```python
from build123d import *

# Parameters (mm, degrees)
SKETCH1_R                = 28.5
BOSS_EXTRUDE1_DEPTH      = 3
BOSS_EXTRUDE4_DEPTH      = 20
BOSS_EXTRUDE7_DEPTH      = 3
SKETCH7_R                = 27
SKETCH7_R_2              = 25
CUT_EXTRUDE1_DEPTH       = 3
CUT_EXTRUDE2_START       = -5
CUT_EXTRUDE2_DEPTH       = 5
CUT_EXTRUDE3_START       = -5
CUT_EXTRUDE3_DEPTH       = 5
BOSS_EXTRUDE8_DEPTH      = 2
BOSS_EXTRUDE8_DEPTH_BACK = 0.5
SKETCH10_R               = 26.875
CHAMFER1_SIZE            = 13.49895933
BOSS_EXTRUDE9_START      = 8
SKETCH11_R               = 26.875
SKETCH11_R_2             = 25.125
BOSS_EXTRUDE9_DEPTH      = 8
CUT_EXTRUDE4_START       = -2
CUT_EXTRUDE4_DEPTH       = 2
SKETCH12_R               = 5
BOSS_EXTRUDE10_DEPTH     = 6
CUT_EXTRUDE5_DEPTH       = 6


with BuildPart() as part:
    # Sketch1 → Boss-Extrude1 (new body)
    with BuildSketch(Plane(origin=(0, 0, 0), x_dir=(1, 0, 0), z_dir=(0, 1, 0))):
        with Locations(Location((0, 0, 0), (0, 0, 270))):
            Circle(SKETCH1_R)
    extrude(amount=BOSS_EXTRUDE1_DEPTH)

    # Sketch2 → Boss-Extrude4 (add)
    with BuildSketch(Plane(origin=(0, 3, 0), x_dir=(1, 0, 0), z_dir=(0, 1, 0))):
        with BuildLine():
            Line((-9, -20.223805295), (-9, -18.723805295))
            ThreePointArc((-9, -18.723805295), (-11.855740218, -15.445899804), (-13.568253388, -11.45))
            ThreePointArc((-13.568253388, -11.45), (-14, -8), (-13.568253388, -4.55))
            ThreePointArc((-13.568253388, -4.55), (0, 6), (13.568253388, -4.55))
            ThreePointArc((13.568253388, -4.55), (14, -8), (13.568253388, -11.45))
            ThreePointArc((13.568253388, -11.45), (11.855740218, -15.445899804), (9, -18.723805295))
            Line((9, -18.723805295), (9, -20.223805295))
            Line((9, -20.223805295), (7.35, -22))
            Line((7.35, -22), (7.617272727, -27.463196394))
            ThreePointArc((7.617272727, -27.463196394), (22.686364547, -17.250474302), (28.5, 0))
            ThreePointArc((28.5, 0), (-17.250474302, 22.686364547), (-7.617272727, -27.463196394))
            Line((-7.617272727, -27.463196394), (-7.35, -22))
            Line((-7.35, -22), (-9, -20.223805295))
        make_face()
    extrude(amount=BOSS_EXTRUDE4_DEPTH)

    # Boss-Extrude7: read off the stored shape, not the designer's step
    # Boss-Extrude7 outline → Boss-Extrude7 (add)
    with BuildSketch(Plane(origin=(0, 23, 0), x_dir=(1, 0, 0), z_dir=(0, 1, 0))):
        with BuildLine():
            ThreePointArc((7.617272727, -27.463196394), (0, 28.5), (-7.617272727, -27.463196394))
            Line((-7.617272727, -27.463196394), (-7.542031899, -25.92523394))
            ThreePointArc((-7.542031899, -25.92523394), (0, 27), (7.542031899, -25.92523394))
            Line((7.542031899, -25.92523394), (7.617272727, -27.463196394))
        make_face()
        with BuildLine():
            ThreePointArc((7.441330866, -23.866851383), (0, 25), (-7.441330866, -23.866851383))
            Line((-7.441330866, -23.866851383), (-7.365455329, -22.315915124))
            ThreePointArc((-7.365455329, -22.315915124), (0, 23.5), (7.365455329, -22.315915124))
            Line((7.365455329, -22.315915124), (7.441330866, -23.866851383))
        make_face()
    extrude(amount=BOSS_EXTRUDE7_DEPTH)

    # Sketch7 → Cut-Extrude1 (cut)
    with BuildSketch(Plane.XZ):
        with Locations(Location((0, 0, 0), (0, 0, 270))):
            Circle(SKETCH7_R)
        with Locations(Location((0, 0, 0), (0, 0, 270))):
            Circle(SKETCH7_R_2, mode=Mode.SUBTRACT)
    extrude(amount=-CUT_EXTRUDE1_DEPTH, mode=Mode.SUBTRACT)

    # Sketch8 → Cut-Extrude2 (cut)
    with BuildSketch(Plane(origin=(0, 3, 0), x_dir=(1, 0, 0), z_dir=(0, 1, 0)).offset(CUT_EXTRUDE2_START)):
        with BuildLine():
            Line((-7.542031899, -25.92523394), (-7.617272727, -27.463196394))
            ThreePointArc((-7.617272727, -27.463196394), (0, -28.5), (7.617272727, -27.463196394))
            Line((7.617272727, -27.463196394), (7.542031899, -25.92523394))
            ThreePointArc((7.542031899, -25.92523394), (0, -27), (-7.542031899, -25.92523394))
        make_face()
    extrude(amount=CUT_EXTRUDE2_DEPTH, mode=Mode.SUBTRACT)

    # Sketch9 → Cut-Extrude3 (cut)
    with BuildSketch(Plane(origin=(0, 3, 0), x_dir=(1, 0, 0), z_dir=(0, 1, 0)).offset(CUT_EXTRUDE3_START)):
        with BuildLine():
            Line((-7.35, -22), (-7.441330866, -23.866851383))
            ThreePointArc((-7.441330866, -23.866851383), (0, -25), (7.441330866, -23.866851383))
            Line((7.441330866, -23.866851383), (7.35, -22))
            Line((7.35, -22), (9, -20.223805295))
            Line((9, -20.223805295), (9, -18.723805295))
            ThreePointArc((9, -18.723805295), (0, 6), (-9, -18.723805295))
            Line((-9, -18.723805295), (-9, -20.223805295))
            Line((-9, -20.223805295), (-7.35, -22))
        make_face()
    extrude(amount=CUT_EXTRUDE3_DEPTH, mode=Mode.SUBTRACT)

    # Sketch10 → Boss-Extrude8 (add, two sides: drawn at the far end of the back side and taken through both)
    with BuildSketch(Plane.XY.offset(27.463196394).offset(-BOSS_EXTRUDE8_DEPTH_BACK)):
        with Locations((0, 13)):
            Circle(SKETCH10_R)
    extrude(amount=BOSS_EXTRUDE8_DEPTH + BOSS_EXTRUDE8_DEPTH_BACK)

    # Chamfer1
    # the kernel refuses this chamfer: 13.49895933, 12 mm, written as the material it adds along each edge
    with BuildSketch(Plane(origin=(9.23233666, 23, 26.963196394), x_dir=(0.8582935658681564, 0, -0.5131589956235051), z_dir=(0, -1, 0))) as chamfer1_piece_1:
        with BuildLine():
            Line((11.824703255, 0), (CHAMFER1_SIZE * 0.85829356586, CHAMFER1_SIZE * 0.513158995619))
            Line((CHAMFER1_SIZE * 0.85829356586, CHAMFER1_SIZE * 0.513158995619), (0, 0))
            ThreePointArc((0, 0), (5.921946236, 0.620003797), (11.824703255, 0))
        make_face()
    extrude(amount=23)
    with BuildSketch(Plane(origin=(-9.23233666, 23, 26.963196394), x_dir=(-0.8582935658681565, 0, -0.5131589956235051), z_dir=(0, -1, 0))) as chamfer1_piece_2:
        with BuildLine():
            Line((11.824703255, 0), (CHAMFER1_SIZE * 0.85829356586, -CHAMFER1_SIZE * 0.513158995619))
            Line((CHAMFER1_SIZE * 0.85829356586, -CHAMFER1_SIZE * 0.513158995619), (0, 0))
            ThreePointArc((0, 0), (5.921946236, -0.620003797), (11.824703255, 0))
        make_face()
    extrude(amount=23)
    with BuildSketch(Plane(origin=(-9.232336658, 26, 26.963196394), x_dir=(-0.8582935658951355, 0, -0.5131589955783807), z_dir=(0, -1, 0))) as chamfer1_piece_3:
        with BuildLine():
            Line((11.824703255, 0), (CHAMFER1_SIZE * 0.858293565887, -CHAMFER1_SIZE * 0.513158995574))
            Line((CHAMFER1_SIZE * 0.858293565887, -CHAMFER1_SIZE * 0.513158995574), (0, 0))
            ThreePointArc((0, 0), (5.921946236, -0.620003797), (11.824703255, 0))
        make_face()
    extrude(amount=3)
    with BuildSketch(Plane(origin=(9.232336658, 26, 26.963196394), x_dir=(0.8582935658951357, 0, -0.5131589955783805), z_dir=(0, -1, 0))) as chamfer1_piece_4:
        with BuildLine():
            Line((11.824703255, 0), (CHAMFER1_SIZE * 0.858293565887, CHAMFER1_SIZE * 0.513158995574))
            Line((CHAMFER1_SIZE * 0.858293565887, CHAMFER1_SIZE * 0.513158995574), (0, 0))
            ThreePointArc((0, 0), (5.921946236, 0.620003797), (11.824703255, 0))
        make_face()
    extrude(amount=3)

    # Sketch11 → Boss-Extrude9 (add)
    with BuildSketch(Plane.XY.offset(29.463196394).offset(BOSS_EXTRUDE9_START)):
        with Locations((0, 13)):
            Circle(SKETCH11_R)
        with Locations((0, 13)):
            Circle(SKETCH11_R_2, mode=Mode.SUBTRACT)
    extrude(amount=-BOSS_EXTRUDE9_DEPTH)

    # Sketch13 → Cut-Extrude4 (cut)
    with BuildSketch(Plane(origin=(0, 23, 0), x_dir=(1, 0, 0), z_dir=(0, 1, 0)).offset(CUT_EXTRUDE4_START)):
        with BuildLine():
            Line((13.568253388, -11.45), (17.5, -11.45))
            ThreePointArc((17.5, -11.45), (20.95, -8), (17.5, -4.55))
            Line((17.5, -4.55), (13.568253388, -4.55))
            ThreePointArc((13.568253388, -4.55), (0, 6), (-13.568253388, -4.55))
            Line((-13.568253388, -4.55), (-17.5, -4.55))
            ThreePointArc((-17.5, -4.55), (-20.95, -8), (-17.5, -11.45))
            Line((-17.5, -11.45), (-13.568253388, -11.45))
            ThreePointArc((-13.568253388, -11.45), (-11.855740218, -15.445899804), (-9, -18.723805295))
            Line((-9, -18.723805295), (-9, -20.223805295))
            Line((-9, -20.223805295), (-7.35, -22))
            Line((-7.35, -22), (-7.35, -25))
            Line((-7.35, -25), (7.35, -25))
            Line((7.35, -25), (7.35, -22))
            Line((7.35, -22), (9, -20.223805295))
            Line((9, -20.223805295), (9, -18.723805295))
            ThreePointArc((9, -18.723805295), (11.855740218, -15.445899804), (13.568253388, -11.45))
        make_face()
    extrude(amount=CUT_EXTRUDE4_DEPTH, mode=Mode.SUBTRACT)

    # Sketch12 → Boss-Extrude10 (add)
    with BuildSketch(Plane.XY.offset(29.463196394)):
        with Locations((0, 13)):
            Circle(SKETCH12_R)
    extrude(amount=BOSS_EXTRUDE10_DEPTH)

    # Sketch14 → Cut-Extrude5 (cut)
    with BuildSketch(Plane.XY.offset(35.463196394)):
        with BuildLine():
            Line((-1.322875656, 11.5), (1.322875656, 11.5))
            ThreePointArc((1.322875656, 11.5), (2, 13), (1.322875656, 14.5))
            Line((1.322875656, 14.5), (-1.322875656, 14.5))
            ThreePointArc((-1.322875656, 14.5), (-2, 13), (-1.322875656, 11.5))
        make_face()
    extrude(amount=-CUT_EXTRUDE5_DEPTH, mode=Mode.SUBTRACT)


solid = part.part
```
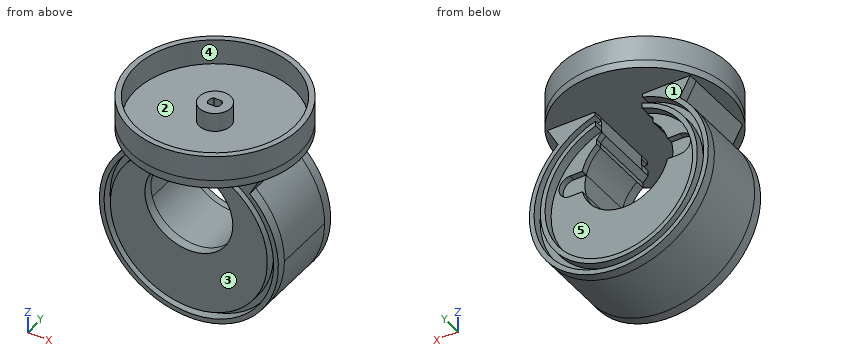
Check sheet for the modelled part. Datum: model origin and axes. Units: mm. Face numbers are marked on the shaded views. A direction names the side the tool comes from. Round coordinates to 2 decimals unless told otherwise and drop trailing zeros. Loops run counter-clockwise (first coordinate to the right, second up) from the corner with the lowest first, then second, coordinate; pieces in that order, holes last. Notation, with made-up numbers: M 16,-35 L 51,-35 A24 cw 51,-2 Z; hole C 18,65.5 d3. An arc over 180 degrees is marked long. Answer as a JSON object with one key per item and string values.
1. Scan lines: line 1 (Y direction, x = 0, z = 35.75) (3 decimals); line 2 (Y direction, x = 0, z = 34) (3 decimals); line 3 (X direction, y = 24.4, z = 0). Record each from-to range of solid material in increasing order.
Reply:
{"line 1": "y = -13.875 to -12.125, 38.125 to 39.875", "line 2": "y = -13.875 to -12.125, 8 to 11.5, 14.5 to 18, 38.125 to 39.875", "line 3": "x = -28.5 to -27, -25 to -23.5, 23.5 to 25, 27 to 28.5"}
2. Access from +Z, -Z, +X, -X, +Y, -Y to the whole of each face (thin tool, end or side, straight path). Record for the marked faces 1 and 2.
Reply:
{"face 1": "-Z, +X, -X, +Y", "face 2": "+Z"}
3. Gauge pin test, flat ends, axial feed: P1, Ø1, axis at x = 15.5, y = 22.5, coming from the +Z side; P2, Ø8, axis at y = 4.5, z = 30, coming from the -X side; P3, Ø6, axis at x = -10, z = 12, coming from the +Y side; P4, Ø2, axis at x = 18, z = 7, coming from the +Y side. Record the tip position at first contact, or that the pin passes through.
Reply:
{"P1": "stops at z = 29.46", "P2": "stops at x = -26.5", "P3": "passes through", "P4": "stops at y = 21"}
4. Section check A-A (x = -6). Record the boundary of the cut face in (y, z), plus the area to 3 significant figures.
Reply:
{"outline": "M -13.2,26.96 L 39.2,26.96 L 39.2,37.46 L 37.4,37.46 L 37.4,29.46 L -11.4,29.46 L -11.4,37.46 L -13.2,37.46 Z; M 0,-27.86 L 26,-27.86 L 26,-26.32 L 23,-26.32 L 23,-24.27 L 26,-24.27 L 26,-22.72 L 23,-22.72 L 23,-4.65 L 0,-4.65 L 0,-24.27 L 3,-24.27 L 3,-26.32 L 0,-26.32 Z", "area": "697 mm²"}
5. Section check D-D (z = -10.5). Record the boundary of the cut face in (x, y), plus the area to 3 significant figures.
Reply:
{"outline": "M -26.5,0 L -24.87,0 L -24.87,3 L -22.69,3 L -22.69,0 L 22.69,0 L 22.69,3 L 24.87,3 L 24.87,0 L 26.5,0 L 26.5,26 L 24.87,26 L 24.87,23 L 22.69,23 L 22.69,26 L 21.02,26 L 21.02,23 L -21.02,23 L -21.02,26 L -22.69,26 L -22.69,23 L -24.87,23 L -24.87,26 L -26.5,26 Z", "area": "1,230 mm²"}
6. Section check B-B (y = 13). Record the boundary of the cut face in (x, z) (3 decimals).
Reply:
{"outline": "M -26.875,26.963 L -22.731,26.963 L -19.381,20.895 A28.5 ccw long 19.381,20.895 L 22.731,26.963 L 26.875,26.963 L 26.875,37.463 L 25.125,37.463 L 25.125,29.463 L 5,29.463 L 5,35.463 L 2,35.463 L 2,29.463 L -2,29.463 L -2,35.463 L -5,35.463 L -5,29.463 L -25.125,29.463 L -25.125,37.463 L -26.875,37.463 Z; hole M -9,18.724 A14 ccw long 9,18.724 L 9,20.224 L 7.35,22 L 7.593,26.963 L -7.593,26.963 L -7.35,22 L -9,20.224 Z"}
7. Mould release check, pull along X, two halves, no side actions. Record for the marked faces 3, 4 and 5: pulls with the +X half, pulls with the -X half, needs draft (parallel to the pull), parting line crosses it, or undercut.
Reply:
{"face 3": "needs draft", "face 4": "undercut", "face 5": "undercut"}
